from build123d import *

# Parameters (mm, degrees)
ESQUISSE1_R             = 2.5
BOSS_EXTRU_1_DEPTH      = 4
ESQUISSE2_R             = 2.1
ESQUISSE2_R_2           = 2
ENL_V_MAT_EXTRU_1_DEPTH = 4
BOSS_EXTRU_2_DEPTH      = 6
CONG_1_R                = 2


with BuildPart() as part:
    # Esquisse1 → Boss.-Extru.1 (new body)
    with BuildSketch(Plane(origin=(0, 0, 0), x_dir=(1, 0, 0), z_dir=(0, 1, 0))):
        Polygon((0, 218), (0, 186), (9, 186), (9, 159), (-41, 129), (-41, 89), (9, 59), (9, 32), (0, 32), (0, 0), (32, 0), (32, 9), (186, 9), (186, 0), (218, 0), (218, 32), (209, 32), (209, 186), (218, 186), (218, 218), (186, 218), (186, 209), (159, 209), (129, 259), (89, 259), (59, 209), (32, 209), (32, 218), align=None)
        with Locations(Location((8, 210, 0), (0, 0, 270))):
            Circle(ESQUISSE1_R, mode=Mode.SUBTRACT)
        with Locations(Location((210, 210, 0), (0, 0, 270))):
            Circle(ESQUISSE1_R, mode=Mode.SUBTRACT)
        with Locations(Location((210, 8, 0), (0, 0, 270))):
            Circle(ESQUISSE1_R, mode=Mode.SUBTRACT)
        with Locations(Location((8, 8, 0), (0, 0, 270))):
            Circle(ESQUISSE1_R, mode=Mode.SUBTRACT)
    extrude(amount=BOSS_EXTRU_1_DEPTH)

    # Esquisse2 → Enlèv. mat.-Extru.1 (cut)
    with BuildSketch(Plane(origin=(0, 4, 0), x_dir=(1, 0, 0), z_dir=(0, 1, 0))):
        with Locations(Location((172.5, 22.6, 0), (0, 0, 90))):
            Circle(ESQUISSE2_R)
        with Locations(Location((153, 82, 0), (0, 0, 90))):
            Circle(ESQUISSE2_R)
        with Locations(Location((20, 107, 0), (0, 0, 90))):
            Circle(ESQUISSE2_R)
        with Locations(Location((49, 122.5, 0), (0, 0, 270))):
            Circle(ESQUISSE2_R_2)
        with Locations(Location((144, 122.5, 0), (0, 0, 270))):
            Circle(ESQUISSE2_R_2)
        with Locations(Location((144, 145, 0), (0, 0, 270))):
            Circle(ESQUISSE2_R_2)
        with Locations(Location((49, 145, 0), (0, 0, 270))):
            Circle(ESQUISSE2_R_2)
        with Locations(Location((67.6, 199.5, 0), (0, 0, 270))):
            Circle(ESQUISSE2_R_2)
        with Locations(Location((67.6, 150.9, 0), (0, 0, 270))):
            Circle(ESQUISSE2_R_2)
        with Locations(Location((125.4, 150.9, 0), (0, 0, 90))):
            Circle(ESQUISSE2_R_2)
        with Locations(Location((125.4, 199.5, 0), (0, 0, 90))):
            Circle(ESQUISSE2_R_2)
    extrude(amount=-ENL_V_MAT_EXTRU_1_DEPTH, mode=Mode.SUBTRACT)

    # Esquisse4 → Boss.-Extru.2 (add)
    with BuildSketch(Plane(origin=(0, 4, 0), x_dir=(1, 0, 0), z_dir=(0, 1, 0))):
        Polygon((198.7, 14.3), (183.7, 14.3), (183.7, 19.3), (196.353215425, 19.3), (198.7, 21.646784575), (198.7, 34.3), (203.7, 34.3), (203.7, 19.3), align=None)
        Polygon((19.3, 203.7), (34.3, 203.7), (34.3, 198.7), (21.646784575, 198.7), (19.3, 196.353215425), (19.3, 183.7), (14.3, 183.7), (14.3, 198.7), align=None)
        Polygon((203.7, 198.7), (203.7, 183.7), (198.7, 183.7), (198.7, 196.353215425), (196.353215425, 198.7), (183.7, 198.7), (183.7, 203.7), (198.7, 203.7), align=None)
    extrude(amount=BOSS_EXTRU_2_DEPTH)

    # Congé1
    cong_1_edges = [part.edges().sort_by_distance(p)[0] for p in [
        (0, 2, 0),
        (0, 2, -32),
        (9, 2, -59),
        (-41, 2, -89),
        (-41, 2, -129),
        (9, 2, -159),
        (9, 2, -186),
        (0, 2, -186),
        (0, 2, -218),
        (32, 2, -218),
        (32, 2, -209),
        (59, 2, -209),
        (89, 2, -259),
        (129, 2, -259),
        (159, 2, -209),
        (186, 2, -209),
        (186, 2, -218),
        (218, 2, -218),
        (218, 2, -186),
        (209, 2, -186),
        (209, 2, -32),
        (218, 2, -32),
        (218, 2, 0),
        (186, 2, 0),
        (186, 2, -9),
        (32, 2, -9),
        (32, 2, 0),
    ]]
    fillet(cong_1_edges, radius=CONG_1_R)


solid = part.part
Read the model definition and answer for the solid it produces. Units are mm, in the model's axes. A direction names the side the tool comes from. Round coordinates to 2 decimals unless told otherwise and drop trailing zeros. Write each loop counter-clockwise with the first axis right and the second up, starting at its lowest first coordinate (ties: lowest second). Pieces come first, ordered by that corner, then holes.
1. The part is cut by section A-A, the plane y = 7.75. Determine the outline of the cut face in (x, z).
2. Which of the six approach directions +Z, -Z, +X, -X, +Y, -Y give full straight-line access (tool end or side, diameter ignored) to faces 4 (the face through (-16, 2, -144)), 5 (the face through (191, 7, -203.7)), 6 (the face through (28, 7, -198.7)), 7 (the face through (190, 7, -19.3))?
3. Determine the mould class of faces 1 (the face through (20, 10, -198)), 2 (the face through (198.7, 7, -28)), 3 (the face through (190, 7, -198.7)) for opening direction X: pulls with the +X half, pulls with the -X half, needs draft (parallel to the pull), parting line crosses it, or undercut.
4. The part is cut by section B-B, the plane z = -232.5. Determine the outline of the cut face in (x, y).
5. Straight lines are drawn through the part: L1, parallel to X at y = 1.6, z = -199.5; L2, parallel to X at y = 2.85, z = -145; L3, parallel to Z at x = 20, y = 1.9. For each, find the intervals that lie inside material, in ascending order.
6. Given pin 1 Ø3 at (x, y) = (214, 2) entering from -Z; pin 2 Ø1.2 at (y, z) = (2.5, -48) entering from -X; pin 3 Ø2.5 at (x, z) = (144, -122.5) entering from -Y; pin 4 Ø2 at (y, z) = (3.5, -178.5) entering from +X, each flat-ended and moving along its own axis, determine where each tip first touches the part or whether it passes through.
7. The part is cut by section C-C, the plane z = -169. Determine the outline of the cut face in (x, y), then the cut area to 3 significant figures.
Values:
1. outline: (14.3, -198.7) - (19.3, -203.7) - (34.3, -203.7) - (34.3, -198.7) - (21.65, -198.7) - (19.3, -196.35) - (19.3, -183.7) - (14.3, -183.7) - close; (183.7, -203.7) - (198.7, -203.7) - (203.7, -198.7) - (203.7, -183.7) - (198.7, -183.7) - (198.7, -196.35) - (196.35, -198.7) - (183.7, -198.7) - close; (183.7, -19.3) - (196.35, -19.3) - (198.7, -21.65) - (198.7, -34.3) - (203.7, -34.3) - (203.7, -19.3) - (198.7, -14.3) - (183.7, -14.3) - close
2. face 4: -X, +Y, -Y
2. face 5: -Z, +X, -X, +Y
2. face 6: +Z, +Y
2. face 7: -X, +Y
3. face 1: needs draft
3. face 2: pulls with the -X half
3. face 3: undercut
4. outline: (73.1, 0) - (144.9, 0) - (144.9, 4) - (73.1, 4) - close
5. L1: x = 0 to 65.6, 69.6 to 123.4, 127.4 to 218
5. L2: x = -14.33 to 47, 51 to 142, 146 to 209
5. L3: z = -218 to -109.1, -104.9 to 0
6. pin 1: stops at z = -218
6. pin 2: stops at x = 9
6. pin 3: passes through
6. pin 4: stops at x = 209
7. outline: (9, 0) - (209, 0) - (209, 4) - (9, 4) - close
7. area: 800 mm2
